```python
from build123d import *

# Parameters (mm, degrees)
SKETCH3_W           = 96
SKETCH3_H           = 20
BOSS_EXTRUDE1_DEPTH = 270
SHELL1_T            = -4


with BuildPart() as part:
    # Sketch3 → Boss-Extrude1 (new body)
    with BuildSketch(Plane.XY):
        with Locations((48, 10)):
            Rectangle(SKETCH3_W, SKETCH3_H)
    extrude(amount=-BOSS_EXTRUDE1_DEPTH)

    # Shell1
    shell1_openings = [part.faces().sort_by_distance(p)[0] for p in [
        (48, 20, -135),
    ]]
    offset(amount=SHELL1_T, openings=shell1_openings, kind=Kind.INTERSECTION)


solid = part.part
```
Input: part model. Units: mm. Frame: model coordinates. A direction names the side the tool comes from. Coordinates: 2 decimals unless noted, no trailing zeros. Write each loop counter-clockwise with the first axis right and the second up, starting at its lowest first coordinate (ties: lowest second). Pieces come first, ordered by that corner, then holes.
1) Mould query, pull axis Z, two halves, no side actions, for faces 1 (the flat face through (4, 12, -133)), 2 (the flat face through (0, 10, -133)), 3 (the flat face through (47, 10, -270)). Classes: pulls with the +Z half, pulls with the -Z half, needs draft (parallel to the pull), parting line crosses it, or undercut.
2) Section C-C on z = -128. Output: boundary loops of the cut face in (x, y), and give its area (3 significant figures).
3) Set-up query: faces 4 (the flat face through (47, 4, -133)), 5 (the flat face through (47, 0, -133)). Return all of +Z, -Z, +X, -X, +Y, -Y with unobstructed straight access to the full face (end or side cutting, diameter ignored); none if empty.
4) Section A-A on y = 16.5. Output: boundary loops of the cut face in (x, z).
5) Section B-B on x = 37.5. Output: boundary loops of the cut face in (y, z), and give its area (3 significant figures).
6) Material intervals for line 1 along X through (y, z) = (14, -58); line 2 along Z through (x, y) = (58, 12); line 3 along Y through (x, z) = (63.5, -206), sorted ascending.
7) Pin query (flat end, axial travel): pin 1 Ø5 at (x, z) = (29, -62.5) entering from -Y; pin 2 Ø1 at (x, z) = (20.5, -185) entering from +Y. Return the tip coordinate at first contact, or that it passes through.
Check result:
1. face 1: undercut
1. face 2: needs draft
1. face 3: pulls with the -Z half
2. outline: (0, 0) - (96, 0) - (96, 20) - (92, 20) - (92, 4) - (4, 4) - (4, 20) - (0, 20) - close
2. area: 512 mm2
3. face 4: +Y
3. face 5: +Z, -Z, +X, -X, -Y
4. outline: (0, -270) - (96, -270) - (96, 0) - (0, 0) - close; hole (4, -266) - (92, -266) - (92, -4) - (4, -4) - close
5. outline: (0, -270) - (20, -270) - (20, -266) - (4, -266) - (4, -4) - (20, -4) - (20, 0) - (0, 0) - close
5. area: 1,210 mm2
6. line 1: x = 0 to 4, 92 to 96
6. line 2: z = -270 to -266, -4 to 0
6. line 3: y = 0 to 4
7. pin 1: stops at y = 0
7. pin 2: stops at y = 4
